Autodesk Inventor part; units mm, degrees
ref_plane "YZ Plane" through (0, 0, 0) normal (1, 0, 0) x (0, 1, 0)
ref_plane "XZ Plane" through (0, 0, 0) normal (0, 1, 0) x (-1, 0, 0)
ref_plane "XY Plane" through (0, 0, 0) normal (0, 0, 1) x (1, 0, 0)
sketch "Sketch2" plane through (0, 0, 0) normal (0, 1, 0) x (-1, 0, 0)
  line L0 (-0.1126, -21.6377) -> (12.3874, -21.6377)
  line L1 (-0.1126, -21.6377) -> (-12.6126, -21.6377)
  line L2 (12.3874, -21.6377) -> (24.8874, 0.0129)
  line L3 (24.8874, 0.0129) -> (12.3874, 21.6635)
  line L4 (12.3874, 21.6635) -> (-12.6126, 21.6635)
  line L5 (-12.6126, 21.6635) -> (-25.1126, 0.0129)
  line L6 (-25.1126, 0.0129) -> (-12.6126, -21.6377)
  point P0 (0, 0)
  dimension "d12" = 12.5
  dimension "d13" = 12.5
  dimension "d14" = 25
  dimension "d15" = 25
  dimension "d16" = 120
  dimension "d17" = 25
  dimension "d18" = 25
  dimension "d19" = 120
extrude "Extrusion2" add sketch "Sketch2" along normal blind 50
shell "Shell1" thickness 5 removed faces 1 at (0.1126, 0, 7.2298)
sketch "Sketch3" plane through (-12.3874, 0, 21.6635) normal (0, 0, 1) x (1, 0, 0)
  line L0 (7.5, 25.4958) -> (17.5, 25.4958)
  line L1 (17.5, 25.4958) -> (17.5, -0.0042)
  line L2 (17.5, -0.0042) -> (7.5, -0.0042)
  line L3 (7.5, -0.0042) -> (7.5, 25.4958)
  line L4 (0, 0) -> (0, 50)
  point P0 (12.3874, 0)
  dimension "d23" = 25.5
  dimension "d24" = 10
  dimension "d25" = 7.5
extrude "Extrusion3" cut sketch "Sketch3" against normal blind 5
sketch "Sketch4" plane through (12.6126, 0, -21.6377) normal (0.8660254, 0, -0.5) x (-0.5, 0, -0.8660254)
  line L0 (-17.5, 25.4905) -> (-7.5, 25.4905)
  line L1 (-7.5, 25.4905) -> (-7.5, -0.0095)
  line L2 (-7.5, -0.0095) -> (-17.5, -0.0095)
  line L3 (-17.5, -0.0095) -> (-17.5, 25.4905)
  line L4 (-25, 0) -> (-25, 50)
  point P0 (-12.4325, 0)
  point P1 (12.3874, 0)
  dimension "d28" = 25.5
  dimension "d29" = 10
  dimension "d30" = 7.5
extrude "Extrusion4" cut sketch "Sketch4" against normal blind 5
sketch "Sketch5" plane through (-24.8874, 0, 0.0129) normal (-0.8660254, 0, -0.5) x (-0.5, 0, 0.8660254)
  line L0 (-17.5, 25.4996) -> (-7.5, 25.4996)
  line L1 (-7.5, 25.4996) -> (-7.5, -0.0004)
  line L2 (-7.5, -0.0004) -> (-17.5, -0.0004)
  line L3 (-17.5, -0.0004) -> (-17.5, 25.4996)
  line L4 (-25, 0) -> (-25, 50)
  point P0 (-12.4549, 0)
  point P1 (12.3874, 0)
  dimension "d33" = 25.5
  dimension "d34" = 10
  dimension "d35" = 7.5
extrude "Extrusion5" cut sketch "Sketch5" against normal blind 5
sketch "Sketch7" plane through (0, 50, 0) normal (0, 1, 0) x (1, 0, 0)
  circle A0 centre (0, 0) radius 13.5
  dimension "d39" = 27
extrude "Extrusion6" add sketch "Sketch7" along normal blind 10 and the other way blind 15
sketch "Sketch11" plane through (-9.5006, 45, -16.6377) normal (0, -1, 0) x (1, 0, 0)
  line L0 (-9.6132, 16.6506) -> (0, 33.3013)
  line L1 (0, 33.3013) -> (19.2265, 33.3013)
  line L2 (0, 33.3013) -> (19.2265, 33.3013)
  line L3 (19.2265, 33.3013) -> (28.8397, 16.6506)
  line L4 (19.2265, 33.3013) -> (28.8397, 16.6506)
  line L5 (28.8397, 16.6506) -> (19.2265, 0)
  line L6 (28.8397, 16.6506) -> (19.2265, 0)
  line L7 (19.2265, 0) -> (0, 0)
  line L8 (19.2265, 0) -> (0, 0)
  line L9 (0, 0) -> (-9.6132, 16.6506)
  line L10 (-9.6132, 16.6506) -> (0, 33.3013)
  point P0 (9.5006, 16.6377)
extrude "Extrusion8" add sketch "Sketch11" along normal blind 10
sketch "Sketch12" plane through (0, 50, 0) normal (0, 1, 0) x (1, 0, 0)
  line L0 (-12.3874, 21.6377) -> (-24.8874, -0.0129)
  line L1 (25.1126, -0.0129) -> (12.6126, 21.6377)
  line L2 (-12.3874, 21.6377) -> (12.6126, 21.6377)
  line L3 (12.6126, 21.6377) -> (25.1126, -0.0129)
  line L4 (12.6126, -21.6635) -> (25.1126, -0.0129)
  line L5 (25.1126, -0.0129) -> (12.6126, -21.6635)
  line L6 (12.6126, -21.6635) -> (-12.3874, -21.6635)
  line L7 (-24.8874, -0.0129) -> (-12.3874, -21.6635)
  line L8 (-12.3874, -21.6635) -> (-24.8874, -0.0129)
  line L9 (-24.8874, -0.0129) -> (-12.3874, 21.6377)
  point P0 (0, 0)
extrude "Extrusion9" add sketch "Sketch12" along normal blind 10
chamfer "Chamfer1" distance 10 angle 45 1 edges at (0.1126, 60, 21.6635)
chamfer "Chamfer2" distance 10 angle 45 1 edges at (21.7494, 60, 5.8382)
chamfer "Chamfer3" distance 10 angle 45 1 edges at (-21.5241, 60, 5.8382)
chamfer "Chamfer4" distance 10 angle 45 1 edges at (-15.7506, 60, -15.8124)
chamfer "Chamfer5" distance 10 angle 45 1 edges at (5.8861, 60, -21.6377)
chamfer "Chamfer6" distance 10 angle 45 1 edges at (18.8626, 60, -10.8124)
fillet "Fillet9" radius 10 6 edges at (10.2024, 60, 5.8382) (10.2024, 60, -5.8124) (0.1126, 60, -11.6377) (-9.9771, 60, -5.8124) (-9.9771, 60, 5.8382) (0.1126, 60, 11.6635)
hole "Hole2" at (0.1293, 60, 0.1623) direction (0, -1, 0) diameter 3.5 depth 10 tip angle 118
properties part number "center" material "ABS Plastic"
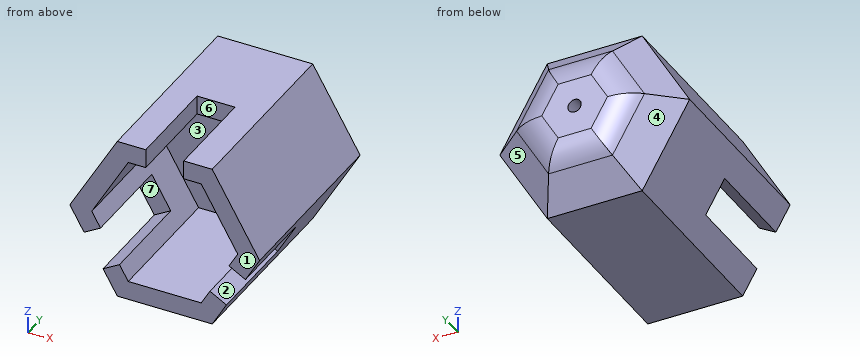
The listing builds one solid part. Answer for the finished solid, in the listing's coordinates (mm). Face numbers are marked on the shaded views. A direction names the side the tool comes from. Give positions to 0.01 mm unless a question says otherwise; leave off trailing zeros. Write each loop counter-clockwise with the first axis right and the second up, starting at its lowest first coordinate (ties: lowest second). Pieces come first, ordered by that corner, then holes.
Item 1: Section B-B, the plane y = 30 is taken. Write down the section's boundary in (x, z), plus the area to 3 significant figures.
Item 2: Section C-C, the plane x = -2.5 is taken. Write down the section's boundary in (y, z), plus the area to 3 significant figures.
Item 3: Which of the six approach directions +Z, -Z, +X, -X, +Y, -Y give full straight-line access (tool end or side, diameter ignored) to the marked faces 5, 6 and 7?
Item 4: Determine the mould class of the marked faces 1, 2, 3 and 4 for opening direction Z: released by +Z, released by -Z, zero draft, split by the parting line, or undercut.
Item 5: Section D-D, the plane z = 18 is taken. Write down the section's boundary in (x, y), plus the area to 3 significant figures.
Item 6: Find the intervals of material crossed by line 1 along Z through (x, y) = (0, 33); line 2 along Z through (x, y) = (3, 15); line 3 along Y through (x, z) = (-15, -3), in increasing order.
Item 7: Flat-ended cylindrical pins translate along their axes: P1, Ø1, axis at x = 9.5, z = -7, coming from the +Y side; P2, Ø10, axis at x = -7.5, z = 8, coming from the -Y side; P3, Ø3, axis at x = -16, z = -7, coming from the -Y side. Find the tip coordinate at first contact, or state that the pin passes through.
Item 8: Section A-A, the plane y = 20 is taken. Write down the section's boundary in (x, z), plus the area to 3 significant figures.
Completed:
1. outline: (-24.89, 0.01) - (-12.39, -21.64) - (12.61, -21.64) - (25.11, 0.01) - (12.61, 21.66) - (-12.39, 21.66) - close; hole (-19.11, 0.01) - (-9.5, -16.64) - (9.73, -16.64) - (19.34, 0.01) - (9.73, 16.66) - (-9.5, 16.66) - close
1. area: 663 mm2
2. outline: (0, -21.64) - (50, -21.64) - (57.07, -14.57) arc R10 ccw to (60, -7.5) - (60, 7.52) arc R10 ccw to (57.07, 14.59) - (50, 21.66) - (25.5, 21.66) - (25.5, 16.66) - (35, 16.66) - (35, -16.64) - (0, -16.64) - close
2. area: 1,200 mm2
3. face 5: -Z, +X, +Y
3. face 6: +Z, -Y
3. face 7: -Y
4. face 1: zero draft
4. face 2: undercut
4. face 3: undercut
4. face 4: released by -Z
5. outline: (-14.5, 0) - (-4.89, 0) - (-4.89, 25.5) - (5.11, 25.5) - (5.11, 0) - (14.73, 0) - (14.73, 50) - (10.5, 53.66) - (-10.27, 53.66) - (-14.5, 50) - close
5. area: 1,300 mm2
6. line 1: z = -21.64 to -16.64, 16.66 to 21.66
6. line 2: z = -21.64 to -16.64
6. line 3: y = 35 to 57.06
7. P1: stops at y = 59.32
7. P2: stops at y = 35
7. P3: stops at y = 25.5
8. outline: (-24.89, 0.01) - (-21.14, -6.48) - (-16.81, -3.98) - (-19.11, 0.01) - (-9.5, 16.66) - (-4.89, 16.66) - (-4.89, 21.66) - (-12.39, 21.66) - close; (-16.14, -15.14) - (-12.39, -21.64) - (12.61, -21.64) - (16.36, -15.14) - (12.03, -12.64) - (9.73, -16.64) - (-9.5, -16.64) - (-11.81, -12.64) - close; (5.11, 16.66) - (9.73, 16.66) - (19.34, 0.01) - (17.03, -3.98) - (21.36, -6.48) - (25.11, 0.01) - (12.61, 21.66) - (5.11, 21.66) - close
8. area: 513 mm2
